Autodesk Inventor part; units mm, degrees
ref_plane "Work Plane1" through (218.6643, -82.569, 72.5272) normal (0, 0, 1) x (1, 0, 0)
ref_plane "YZ Plane" through (0, 0, 0) normal (1, 0, 0) x (0, 1, 0)
ref_plane "XZ Plane" through (0, 0, 0) normal (0, 1, 0) x (-1, 0, 0)
ref_plane "Work Plane1" through (218.6643, -82.569, 72.5272) normal (0, 0, 1) x (1, 0, 0)
sketch "Sketch1" plane through (218.6643, -82.569, 72.5272) normal (0, 0, 1) x (1, 0, 0)
  line L0 (17.0344, 125.1412) -> (87.0344, 125.1412)
  line L1 (87.0344, 125.1412) -> (87.0344, 70.1412)
  line L2 (87.0344, 70.1412) -> (17.0344, 70.1412)
  line L3 (17.0344, 70.1412) -> (17.0344, 125.1412)
  point P0 (-218.6643, 82.569)
  dimension "Floor_Len" = 70
  dimension "Floor_Wid" = 55
extrude "Extrusion1" add sketch "Sketch1" along normal blind 3
sketch "Sketch2" plane through (218.6643, -82.569, 75.5272) normal (0, 0, 1) x (1, 0, 0)
  line L0 (17.0344, 70.1412) -> (87.0344, 70.1412)
  line L1 (87.0344, 125.1412) -> (17.0344, 125.1412)
  line L2 (87.0344, 70.1412) -> (84.0344, 70.1412)
  line L3 (84.0344, 70.1412) -> (84.0344, 125.1412)
  line L4 (84.0344, 125.1412) -> (87.0344, 125.1412)
  line L5 (87.0344, 125.1412) -> (87.0344, 70.1412)
  point P0 (-218.6643, 82.569)
  dimension "Tall_Thick" = 3
extrude "Extrusion2" add sketch "Sketch2" along normal blind 70
sketch "Sketch3" plane through (305.6987, -12.4279, 72.5272) normal (1, 0, 0) x (0, 0, -1)
  line L0 (0, 55) -> (-73, 55)
  line L1 (-73, 0) -> (-73, 55)
  point P0 (72.5272, 12.4279)
  point P1 (-51.5, 27.5)
  dimension "d40" = 21.5
  dimension "d41" = 27.5
hole "Hole1" at (305.6987, 15.0721, 124.0272) direction (-1, 0, 0) diameter 10.5 end through all
sketch "Sketch4" plane through (305.6987, -12.4279, 72.5272) normal (1, 0, 0) x (0, 0, -1)
  circle A0 centre (-51.5, 27.5) radius 5.3956
  circle A1 centre (-51.5, 27.5) radius 5.25
  point P0 (72.5272, 12.4279)
  point P1 (-51.5, 20)
  point P2 (-51.5, 35)
  dimension "d46" = 7.5
  dimension "d47" = 7.5
hole "Hole2" at (305.6987, 7.5721, 124.0272) at (305.6987, 22.5721, 124.0272) direction (-1, 0, 0) diameter 2.5 end through all
sketch "Sketch5" plane through (305.6987, -12.4279, 72.5272) normal (1, 0, 0) x (0, 0, -1)
  circle A0 centre (-51.5, 27.5) radius 5.2922
  circle A1 centre (-51.5, 27.5) radius 5.25
  line L0 (-65.5, 27.5) -> (-44.5, 39.6244)
  line L1 (-44.5, 39.6244) -> (-44.5, 15.3756)
  line L2 (-44.5, 15.3756) -> (-65.5, 27.5)
  point P0 (-65.5, 10)
  point P1 (-65.5, 45)
  point P2 (-26.5, 10)
  point P3 (-26.5, 45)
  dimension "d42" = 14
  dimension "d43" = 17.5
  dimension "d44" = 17.5
  dimension "d45" = 39
hole "Hole3" at (305.6987, -2.4279, 138.0272) at (305.6987, -2.4279, 99.0272) at (305.6987, 32.5721, 99.0272) at (305.6987, 32.5721, 138.0272) at (305.6987, 15.0721, 138.0272) at (305.6987, 2.9478, 117.0272) at (305.6987, 27.1965, 117.0272) direction (-1, 0, 0) diameter 5 end through all
sketch "Sketch6" plane through (242.6987, 66.5721, 72.5272) normal (0, 0, -1) x (0, 1, 0)
  line L0 (-24, -7) -> (-79, -7)
  line L1 (-24, 63) -> (-24, -7)
  point P0 (72.5272, 12.4279)
  point P1 (-51.5, 14.5)
  dimension "d77" = 21.5
  dimension "d78" = 27.5
hole "Hole4" at (257.1987, 15.0721, 72.5272) direction (0, 0, 1) diameter 10.5 end through all
sketch "Sketch7" plane through (270.6987, 15.0721, 72.5272) normal (0, 0, -1) x (-1, 0, 0)
  circle A0 centre (13.5, 0) radius 5.3956
  circle A1 centre (13.5, 0) radius 5.25
  point P0 (72.5272, 12.4279)
  point P1 (13.5, -7.5)
  point P2 (13.5, 7.5)
  dimension "d59" = 7.5
  dimension "d58" = 7.5
hole "Hole5" at (257.1987, 7.5721, 72.5272) at (257.1987, 22.5721, 72.5272) direction (0, 0, 1) diameter 2.5 end through all
sketch "Sketch8" plane through (270.6987, 15.0721, 72.5272) normal (0, 0, -1) x (-1, 0, 0)
  line L0 (35, -27.5) -> (-32, -27.5)
  circle A0 centre (13.5, 0) radius 5.25
  circle A1 centre (13.5, 0) radius 5.25
  line L1 (27.5, 0) -> (6.5, -12.1244)
  line L2 (6.5, -12.1244) -> (6.5, 12.1244)
  line L3 (6.5, 12.1244) -> (27.5, 0)
  point P0 (27.5, 17.5)
  point P1 (27.5, -17.5)
  point P2 (-11.5, 17.5)
  point P3 (-11.5, -17.5)
  dimension "d79" = 17.5
  dimension "d80" = 17.5
  dimension "d82" = 39
  dimension "d83" = 10
  dimension "d84" = 10.5
  dimension "d85" = 14
hole "Hole6" at (243.1987, 15.0721, 72.5272) at (243.1987, 32.5721, 72.5272) at (282.1987, 32.5721, 72.5272) at (282.1987, -2.4279, 72.5272) at (243.1987, -2.4279, 72.5272) at (264.1987, 27.1965, 72.5272) at (264.1987, 2.9478, 72.5272) direction (0, 0, 1) diameter 5 end through all
properties part number "Metal Braket" material "Aluminum 6061"
Could you check a few things on this model? Use its own coordinates, in mm. A direction names the side the tool comes from. Give positions to 0.01 mm unless a question says otherwise; leave off trailing zeros. Order: outer loops, then holes, each group sorted by start corner. A loop starts at its lowest first (then second) coordinate and runs counter-clockwise, first axis right, second up. Notation, with made-up numbers: M 50.5,-7.5 L 96.5,-7.5 A13 ccw 96.5,14.5 Z; hole C 43.5,-27 d1. An arc over 180 degrees is marked long. One line per question, with ' | ' between items.
1. I want a section at A-A (z = 138.5). List the corners of the cut face in (x, y) for me, and give its area (3 significant figures).
Results:
outline: M 302.7,-12.43 L 305.7,-12.43 L 305.7,-4.88 L 302.7,-4.88 Z; M 302.7,0.03 L 305.7,0.03 L 305.7,12.62 L 302.7,12.62 Z; M 302.7,17.53 L 305.7,17.53 L 305.7,30.12 L 302.7,30.12 Z; M 302.7,35.03 L 305.7,35.03 L 305.7,42.57 L 302.7,42.57 Z | area: 121 mm²
2. I want a section at B-B (x = 265.5). List the corners of the cut face in (y, z) for me.
Results:
outline: M -12.43,72.53 L 0.81,72.53 L 0.81,75.53 L -12.43,75.53 Z; M 5.08,72.53 L 25.06,72.53 L 25.06,75.53 L 5.08,75.53 Z; M 29.33,72.53 L 42.57,72.53 L 42.57,75.53 L 29.33,75.53 Z
3. If I drill on line 1 (Z direction, x = 239, y = -1.5); line 2 (X direction, y = 37.5, z = 123.5), over which ranges is the centre line in solid material (lowest first)?
Results:
line 1: 72.53 to 75.53 | line 2: 302.7 to 305.7
4. We'd pull the mould along Y, two halves only. Please class faces 1 (the face through (304.18, 8.33, 125.02)), 2 (the face through (304, 42.572, 93)), 3 (the face through (304, 15, 145.527)): +Y half, -Y half, draft (parallel to the pull), parting line (faces both ways), or undercut.
Results:
face 1: undercut | face 2: +Y half | face 3: draft
5. I'm going to push flat-ended pins straight in: pin 1 (6.5 mm diameter, centred on x = 264.2, y = 2.95, fed in from +Z); pin 2 (10 mm diameter, centred on y = 22, z = 92, fed in from -X); pin 3 (6 mm diameter, centred on y = -2.43, z = 99.03, fed in from +X). Where does each tip first touch, or does it pass through?
Results:
pin 1: z = 75.53 | pin 2: x = 302.7 | pin 3: x = 305.7
6. I want a section at C-C (y = 16.5). List the corners of the cut face in (x, z) for me, and give its area (3 significant figures).
Results:
outline: M 235.7,72.53 L 241.15,72.53 L 241.15,75.53 L 235.7,75.53 Z; M 245.25,72.53 L 252.15,72.53 L 252.15,75.53 L 245.25,75.53 Z; M 262.25,72.53 L 305.7,72.53 L 305.7,118.98 L 302.7,118.98 L 302.7,75.53 L 262.25,75.53 Z; M 302.7,129.08 L 305.7,129.08 L 305.7,135.98 L 302.7,135.98 Z; M 302.7,140.08 L 305.7,140.08 L 305.7,145.53 L 302.7,145.53 Z | area: 335 mm²
7. I want a section at D-D (y = 37.5). List the corners of the cut face in (x, z) for me, and give its area (3 significant figures).
Results:
outline: M 235.7,72.53 L 305.7,72.53 L 305.7,145.53 L 302.7,145.53 L 302.7,75.53 L 235.7,75.53 Z | area: 420 mm²
8. For faces 4 (the face through (269, 15, 75.527)), 5 (the face through (304.178, 32.462, 140.525)), which set-ups out of +Z, -Z, +X, -X, +Y, -Y let a thin tool reach every point of the face, with its end or its side?
Results:
face 4: +Z, -X, +Y, -Y | face 5: +X, -X
